```python
from build123d import *

# Parameters (mm, degrees)
SKETCH_1_W          = 48
SKETCH_1_H          = 20
EXTRUDE_1_DEPTH     = 30
SKETCH_2_W          = 14
SKETCH_2_H          = 30
CUT_EXTRUDE_1_DEPTH = 7
SKETCH_7_W          = 22
SKETCH_7_H          = 30
EXTRUDE_2_DEPTH     = 48
SKETCH_8_W          = 21
SKETCH_8_H          = 30
CUT_EXTRUDE_2_DEPTH = 14
SKETCH_9_W          = 21
SKETCH_9_H          = 30
CUT_EXTRUDE_3_DEPTH = 14
SKETCH_11_W         = 10.4
SKETCH_11_H         = 20.4
CUT_EXTRUDE_4_DEPTH = 56.497747702
SKETCH_13_R         = 4
CUT_EXTRUDE_5_DEPTH = 44.783558558
SKETCH_14_R         = 4
CUT_EXTRUDE_6_DEPTH = 44.783558558
FILLET_1_R          = 7
SKETCH1_W           = 10.4
SKETCH1_H           = 20.4
BOSS_EXTRUDE1_DEPTH = 4
SKETCH_20_R         = 7.5
CUT_EXTRUDE_8_DEPTH = 44.783558558


with BuildPart() as part:
    # Эскиз1 → Бобышка-Вытянуть1 (new body)
    with BuildSketch(Plane(origin=(0, 0, 0), x_dir=(1, 0, 0), z_dir=(0, 1, 0))):
        Rectangle(SKETCH_1_W, SKETCH_1_H)
    extrude(amount=EXTRUDE_1_DEPTH)

    # Эскиз2 → Вырез-Вытянуть1 (cut)
    with BuildSketch(Plane.XY.offset(10)):
        with Locations((0, 15)):
            Rectangle(SKETCH_2_W, SKETCH_2_H)
    extrude(amount=-CUT_EXTRUDE_1_DEPTH, mode=Mode.SUBTRACT)

    # Эскиз7 → Бобышка-Вытянуть2 (add)
    with BuildSketch(Plane(origin=(24, 0, 0), x_dir=(0, 0, -1), z_dir=(1, 0, 0))):
        with Locations((21, 15)):
            Rectangle(SKETCH_7_W, SKETCH_7_H)
    extrude(amount=-EXTRUDE_2_DEPTH)

    # Эскиз8 → Вырез-Вытянуть2 (cut)
    with BuildSketch(Plane(origin=(24, 0, 0), x_dir=(0, 0, -1), z_dir=(1, 0, 0))):
        with Locations((21.5, 15)):
            Rectangle(SKETCH_8_W, SKETCH_8_H)
    extrude(amount=-CUT_EXTRUDE_2_DEPTH, mode=Mode.SUBTRACT)

    # Эскиз9 → Вырез-Вытянуть3 (cut)
    with BuildSketch(Plane.ZY.offset(24)):
        with Locations((-21.5, 15)):
            Rectangle(SKETCH_9_W, SKETCH_9_H)
    extrude(amount=-CUT_EXTRUDE_3_DEPTH, mode=Mode.SUBTRACT)

    # Эскиз11 → Вырез-Вытянуть4 (cut, through all)
    with BuildSketch(Plane.ZY.offset(10)):
        with Locations((-21.5, 15)):
            Rectangle(SKETCH_11_W, SKETCH_11_H)
    extrude(amount=-CUT_EXTRUDE_4_DEPTH, mode=Mode.SUBTRACT)

    # Эскиз13 → Вырез-Вытянуть5 (cut, through all)
    with BuildSketch(Plane(origin=(0, 0, -11), x_dir=(-1, 0, 0), z_dir=(0, 0, -1))):
        with Locations((17, 15)):
            Circle(SKETCH_13_R)
    extrude(amount=-CUT_EXTRUDE_5_DEPTH, mode=Mode.SUBTRACT)

    # Эскиз14 → Вырез-Вытянуть6 (cut, through all)
    with BuildSketch(Plane(origin=(0, 0, -11), x_dir=(-1, 0, 0), z_dir=(0, 0, -1))):
        with Locations((-17, 15)):
            Circle(SKETCH_14_R)
    extrude(amount=-CUT_EXTRUDE_6_DEPTH, mode=Mode.SUBTRACT)

    # Скругление1
    fillet_1_edges = [part.edges().sort_by_distance(p)[0] for p in [
        (-7, 15, 3),
        (7, 15, 3),
    ]]
    fillet(fillet_1_edges, radius=FILLET_1_R - 0.0001)  # a hair under: the kernel refuses the full size

    # Sketch1 → Boss-Extrude1 (add)
    with BuildSketch(Plane(origin=(10, 0, 0), x_dir=(0, 0, -1), z_dir=(1, 0, 0))):
        with Locations((21.5, 15)):
            Rectangle(SKETCH1_W, SKETCH1_H)
    extrude(amount=-BOSS_EXTRUDE1_DEPTH)

    # Эскиз20 → Вырез-Вытянуть8 (cut, through all)
    with BuildSketch(Plane(origin=(0, 0, -11), x_dir=(-1, 0, 0), z_dir=(0, 0, -1))):
        with Locations((-17, 15)):
            Circle(SKETCH_20_R)
        with Locations((17, 15)):
            Circle(SKETCH_20_R)
    extrude(amount=CUT_EXTRUDE_8_DEPTH, mode=Mode.SUBTRACT)


solid = part.part
```
Input: part model. Units: mm. Frame: model coordinates. A direction names the side the tool comes from. Coordinates: 2 decimals unless noted, no trailing zeros. Loops run counter-clockwise (first coordinate to the right, second up) from the corner with the lowest first, then second, coordinate; pieces in that order, holes last. Notation, with made-up numbers: (61, 64) -> (96, 64) arc R10 ccw to (96, 77) -> close; hole circle Ø8 at (7, 80.5). An arc over 180 degrees is marked (long way). Use a Markdown table: item, result.
1) Contact query for flat-ended pins moving along their axis: pin 1 (4 mm diameter, centred on x = 16, y = 19, fed in from -Z); pin 2 (8.5 mm diameter, centred on y = 15.5, z = -22, fed in from -X); pin 3 (6 mm diameter, centred on y = 21.5, z = -25.5, fed in from +X). Output: stop coordinate, or through.
Results found:
| item | result |
|---|---|
| pin 1 | stops at z = -11 |
| pin 2 | stops at x = 6 |
| pin 3 | stops at x = 10 |
2) Cut plane B-B (x = -17). Return the cut outline in (y, z).
Results found:
| item | result |
|---|---|
| outline | (0, -11) -> (11, -11) -> (11, 10) -> (0, 10) -> close; (19, -11) -> (30, -11) -> (30, 10) -> (19, 10) -> close |
3) Cut plane C-C (z = -9). Return the cut outline in (x, y), then the cut area to 3 significant figures.
Results found:
| item | result |
|---|---|
| outline | (-24, 0) -> (24, 0) -> (24, 30) -> (-24, 30) -> close; hole circle Ø8 at (-17, 15); hole circle Ø8 at (17, 15) |
| area | 1,340 mm2 |
4) Cut plane D-D (z = -17). Return the cut outline in (x, y), then the cut area to 3 significant figures.
Results found:
| item | result |
|---|---|
| outline | (-10, 0) -> (10, 0) -> (10, 12.31) arc R7.5 cw to (10, 17.69) -> (10, 30) -> (-10, 30) -> (-10, 25.2) -> (6, 25.2) -> (6, 4.8) -> (-10, 4.8) -> close |
| area | 272 mm2 |
5) Cut plane A-A (y = 15). Give the number of separate pieces and of enclosed holes in the cut face, then the cut area to 3 significant figures.
Results found:
| item | result |
|---|---|
| separate pieces | 3 |
| enclosed holes | 0 |
| area | 833 mm2 |
6) Material intervals for line 1 along Y through (x, z) = (17, 3.25); line 2 along Y through (x, z) = (-6, -23.5); line 3 along X through (y, z) = (14.75, 4.5), sorted ascending. Write a range as from..to.
Results found:
| item | result |
|---|---|
| line 1 | y = 0..11, 19..30 |
| line 2 | y = 0..4.8, 25.2..30 |
| line 3 | x = -24..-20.99, -13.01..-4.33, 4.33..13.01, 20.99..24 |
7) Pull-direction query (Z, two-part tool) for faces 1 (the flat face through (-2, 25.2, -22)), 2 (the flat face through (12, 15, 10)), 3 (the flat face through (10, 6, -21)); classes: released by +Z, released by -Z, zero draft, split by the parting line, or undercut.
Results found:
| item | result |
|---|---|
| face 1 | undercut |
| face 2 | released by +Z |
| face 3 | zero draft |
8) Access query for faces 4 (the flat face through (-10, 27, -22)), 5 (the flat face through (-2, 15, -16.3)), 6 (the cylindrical face through (-9.5, 15, -13.6)). Directions: +Z, -Z, +X, -X, +Y, -Y. A direction counts if a zero-diameter tool reaches every point of the face in a straight line with its end or side. Return the directions, or none.
Results found:
| item | result |
|---|---|
| face 4 | -Z, -X, +Y, -Y |
| face 5 | -X |
| face 6 | -Z, -X |
